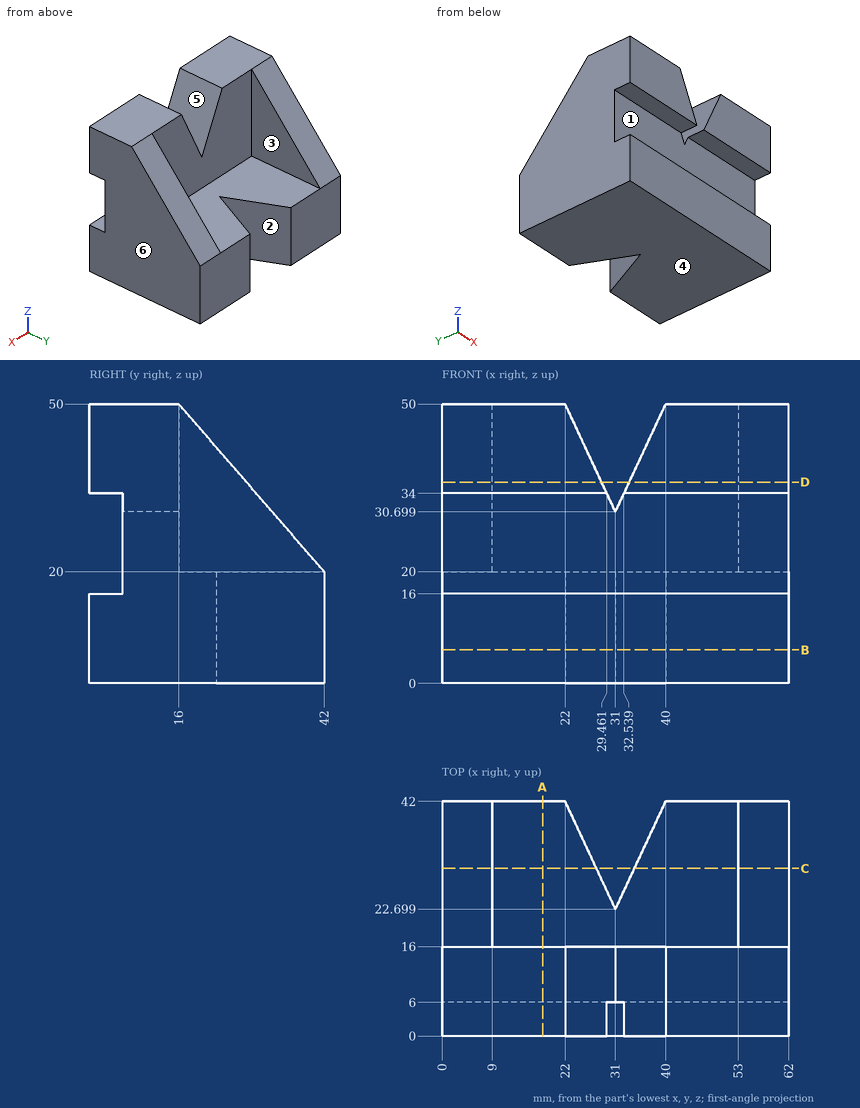
Source: three-view drawing plus pictorial views. Frame: mm from the lowest corner of the part. A direction names the side the tool comes from. Coordinates: 2 decimals unless noted, no trailing zeros. Loops run counter-clockwise (first coordinate to the right, second up) from the corner with the lowest first, then second, coordinate; pieces in that order, holes last. Notation, with made-up numbers: (40, 40.25) -> (82, 40.25) arc R16 ccw to (82, 63.25) -> close; hole circle Ø7 at (15, 8). An arc over 180 degrees is marked (long way). Answer in a Markdown table with one row per item. Add a question column.
Q1. Reachability of the marked faces 1, 2 and 3 from +Z, -Z, +X, -X, +Y, -Y: full face, straight path, thin tool, end or side. Return the list, or none.
Q2. Pull-direction query (X, two-part tool) for the marked faces 4, 5 and 6; classes: pulls with the +X half, pulls with the -X half, needs draft (parallel to the pull), parting line crosses it, or undercut.
Q3. Contact query for flat-ended pins moving along their axis: pin 1 Ø1.5 at (x, y) = (29, 28) entering from +Z; pin 2 Ø14.5 at (x, z) = (36, 23.5) entering from -Y; pin 3 Ø3 at (x, y) = (26.5, 2) entering from +Z (1 decimal). Output: stop coordinate, or through.
Q4. Section D-D on z = 36. Return the cut outline in (x, y).
Q5. Section A-A on x = 18. Return the cut outline in (y, z).
Q6. Ray query, line 1 along X through (y, z) = (34.5, 20.5); line 2 along Y through (x, z) = (25.5, 28); line 3 along Z through (x, y) = (55, 2.5). Return the intervals inside material, ascending.
Q7. Section C-C on y = 30. Return the cut outline in (x, z) (1 decimal), and give its area (3 significant figures).
Q8. Section B-B on z = 6. Return the cut outline in (x, y), and give its area (3 significant figures).
Computed values:
| question | item | result |
|---|---|---|
| 1 | face 1 | +X, -X, -Y |
| 1 | face 2 | +Z, -Z, +Y |
| 1 | face 3 | +Z, +Y |
| 2 | face 4 | needs draft |
| 2 | face 5 | undercut |
| 2 | face 6 | pulls with the +X half |
| 3 | pin 1 | stops at z = 20 |
| 3 | pin 2 | stops at y = 6 |
| 3 | pin 3 | stops at z = 43.6 |
| 4 | outline | (0, 0) -> (28.53, 0) -> (28.53, 16) -> (9, 16) -> (9, 28.13) -> (0, 28.13) -> close; (33.47, 0) -> (62, 0) -> (62, 28.13) -> (53, 28.13) -> (53, 16) -> (33.47, 16) -> close |
| 5 | outline | (0, 0) -> (42, 0) -> (42, 20) -> (16, 20) -> (16, 50) -> (0, 50) -> (0, 34) -> (6, 34) -> (6, 16) -> (0, 16) -> close |
| 6 | line 1 | x = 0 to 9, 53 to 62 |
| 6 | line 2 | y = 6 to 16 |
| 6 | line 3 | z = 0 to 16, 34 to 50 |
| 7 | outline | (0, 0) -> (27.6, 0) -> (27.6, 20) -> (9, 20) -> (9, 33.8) -> (0, 33.8) -> close; (34.4, 0) -> (62, 0) -> (62, 33.8) -> (53, 33.8) -> (53, 20) -> (34.4, 20) -> close |
| 7 | area | 1,350 mm^2 |
| 8 | outline | (0, 0) -> (62, 0) -> (62, 42) -> (40, 42) -> (31, 22.7) -> (22, 42) -> (0, 42) -> close |
| 8 | area | 2,430 mm^2 |
